Geometry check sheet. Reference: the model listing, model coordinates, mm. Face numbers are marked on the shaded views. A direction names the side the tool comes from. Round coordinates to 2 decimals unless told otherwise and drop trailing zeros. Order: outer loops, then holes, each group sorted by start corner. A loop starts at its lowest first (then second) coordinate and runs counter-clockwise, first axis right, second up. Notation, with made-up numbers: (9.25, 83) -> (46.25, 83) arc R11 cw to (46.25, 91) -> close; hole circle Ø5 at (40.5, 27). An arc over 180 degrees is marked (long way). Answer as a JSON object with one key per item and string values. Group by question number.
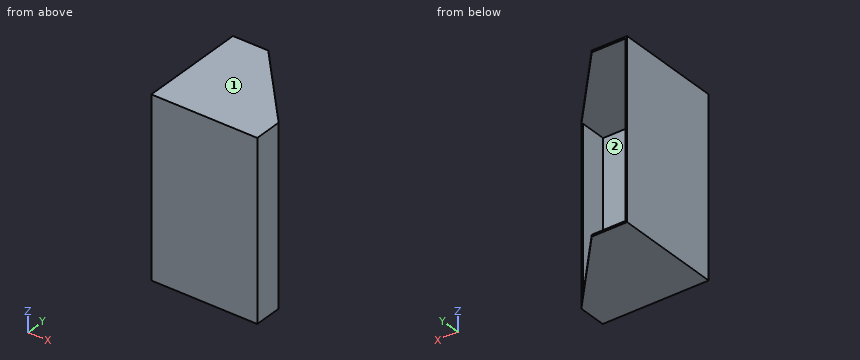
Autodesk Inventor part; units mm, degrees
ref_plane "YZ Plane" through (0, 0, 0) normal (1, 0, 0) x (0, 1, 0)
ref_plane "XZ Plane" through (0, 0, 0) normal (0, 1, 0) x (-1, 0, 0)
ref_plane "XY Plane" through (0, 0, 0) normal (0, 0, 1) x (1, 0, 0)
sketch "Sketch2" plane through (0, 0, 0) normal (0, 1, 0) x (-1, 0, 0)
  line L0 (0, 0) -> (600, 0)
  line L1 (600, 0) -> (600, -1000)
  line L2 (600, -1000) -> (0, -1000)
  line L3 (0, -1000) -> (0, 0)
  dimension "d0" = 600
  dimension "d1" = 1000
extrude "Extrusion1" add sketch "Sketch2" along normal blind 10
sketch "Sketch3" plane through (-600, 0, 0) normal (0, 0, 1) x (1, 0, 0)
  line L0 (600, 10) -> (0, 10)
  line L1 (0, 10) -> (0, 610)
  line L2 (0, 610) -> (200, 610)
  line L3 (200, 610) -> (600, 160)
  line L4 (600, 160) -> (600, 10)
  line L5 (0, 10) -> (600, 10)
  line L6 (600, 160) -> (0, 160) construction
  point P0 (600, 0)
  dimension "d4" = 600
  dimension "d5" = 200
  dimension "d6" = 150
  dimension "d13" = 600
  dimension "d14" = 48.367
extrude "Extrusion2" add sketch "Sketch3" against normal blind 10
ref_plane "Work Plane1" through (0, 0, -500) normal (0, 0, -1) x (-1, 0, 0)
mirror "Mirror1" about plane through (0, 0, -500) normal (0, 0, -1) of "Extrusion2"
sketch "Sketch4" plane through (0, 0, 0) normal (1, 0, 0) x (0, 0, -1)
  line L0 (990, 10) -> (10, 10)
  line L1 (1000, 160) -> (990, 160)
  line L2 (10, 10) -> (990, 10)
  line L3 (990, 10) -> (990, 160)
  line L4 (990, 160) -> (10, 160)
  line L5 (10, 160) -> (10, 10)
  point P0 (0, 0)
extrude "Extrusion3" add sketch "Sketch4" against normal blind 10
sketch "Sketch5" plane through (-600, 0, -1000) normal (-1, 0, 0) x (0, 0, 1)
  line L0 (990, 10) -> (10, 10)
  line L1 (990, 10) -> (990, 610)
  line L2 (10, 10) -> (990, 10)
  line L3 (990, 10) -> (990, 610)
  line L4 (990, 610) -> (10, 610)
  line L5 (10, 610) -> (10, 10)
  point P0 (1000, 0)
extrude "Extrusion4" add sketch "Sketch5" against normal blind 10
properties part number "bois"
Item 1: Sectioned sample at B-B, the plane z = -661.5. Enter the section's corners in (x, y), then the cut area to 3 significant figures.
Item 2: Sectioned sample at A-A, the plane x = -527. Enter the section's corners in (y, z).
Item 3: Depth check by flat-ended pin: pin 1 Ø10 at (y, z) = (323, -714.5) entering from +X; pin 2 Ø3 at (x, z) = (-3, -531.5) entering from +Y. Enter the tip coordinate at first touch or a pass-through.
Item 4: Thickness scan on L1, parallel to Z at x = -263.5, y = 89.5; L2, parallel to Y at x = -293.5, z = -166; L3, parallel to X at y = 264, z = -225.5. Record the ranges inside material, lowest first.
Item 5: Set-up check for the marked faces 1 and 2: record each of +Z, -Z, +X, -X, +Y, -Y from which the full face is reachable in a straight line by a thin tool's end or side.
Result:
{
 "1": {"outline": "(-600, 0) -> (0, 0) -> (0, 160) -> (-10, 160) -> (-10, 10) -> (-590, 10) -> (-590, 610) -> (-600, 610) -> close", "area": "13,500 mm2"},
 "2": {"outline": "(0, -1000) -> (610, -1000) -> (610, -990) -> (10, -990) -> (10, -10) -> (610, -10) -> (610, 0) -> (0, 0) -> close"},
 "3": {"pin 1": "stops at x = -590", "pin 2": "stops at y = 160"},
 "4": {"L1": "z = -1000 to -990, -10 to 0", "L2": "y = 0 to 10", "L3": "x = -600 to -590"},
 "5": {"face 1": "+Z, +X, -X, +Y, -Y", "face 2": "+Y"}
}
